The model under review builds one solid part; all positions refer to its coordinate system, in mm. A direction names the side the tool comes from. Coordinates: 2 decimals unless noted, no trailing zeros. Order: outer loops, then holes, each group sorted by start corner. A loop starts at its lowest first (then second) coordinate and runs counter-clockwise, first axis right, second up. Notation, with made-up numbers: M 13,-39.75 L 38,-39.75 A13 ccw 38,-18.75 Z; hole C -0.5,54 d2. An arc over 180 degrees is marked long. One line per item, written item: value.
```python
from build123d import *

# Parameters (mm, degrees)
MODEL_R             = 1.5
BOSS_EXTRUDE1_DEPTH = 6.6


with BuildPart() as part:
    # Model → Boss-Extrude1 (new body)
    with BuildSketch(Plane.XY):
        with BuildLine():
            Line((3.085786438, -24.814213562), (21.914213562, -5.985786438))
            ThreePointArc((21.914213562, -5.985786438), (22.347759065, -5.33693974), (22.5, -4.571572875))
            Line((22.5, -4.571572875), (22.5, 4.571572875))
            ThreePointArc((22.5, 4.571572875), (22.347759065, 5.33693974), (21.914213562, 5.985786438))
            Line((21.914213562, 5.985786438), (3.085786438, 24.814213562))
            ThreePointArc((3.085786438, 24.814213562), (2.43693974, 25.247759065), (1.671572875, 25.4))
            Line((1.671572875, 25.4), (-16.243953329, 25.4))
            ThreePointArc((-16.243953329, 25.4), (-20.102984306, 23.579289217), (-21.151543558, 19.44315197))
            ThreePointArc((-21.151543558, 19.44315197), (-19.273776994, 0), (-21.151543558, -19.44315197))
            ThreePointArc((-21.151543558, -19.44315197), (-20.102984306, -23.579289217), (-16.243953329, -25.4))
            Line((-16.243953329, -25.4), (1.671572875, -25.4))
            ThreePointArc((1.671572875, -25.4), (2.43693974, -25.247759065), (3.085786438, -24.814213562))
        make_face()
        with Locations((0.385786438, 20.4)):
            Circle(MODEL_R, mode=Mode.SUBTRACT)
        with Locations((0.385786438, -20.4)):
            Circle(MODEL_R, mode=Mode.SUBTRACT)
        with Locations((-7.922562904, 18.5)):
            Circle(MODEL_R, mode=Mode.SUBTRACT)
        with Locations((-7.899139633, -18.5)):
            Circle(MODEL_R, mode=Mode.SUBTRACT)
        with BuildLine():
            Line((-7.5, -2.5527), (7.5, -2.5527))
            ThreePointArc((7.5, -2.5527), (10.0527, 0), (7.5, 2.5527))
            Line((7.5, 2.5527), (-7.5, 2.5527))
            ThreePointArc((-7.5, 2.5527), (-10.0527, 0), (-7.5, -2.5527))
        make_face(mode=Mode.SUBTRACT)
    extrude(amount=BOSS_EXTRUDE1_DEPTH)


solid = part.part
```
(1) We need section D-D, the plane x = 19. State the section outline as (y, z) points.
Geometry results:
outline: M -8.9,0 L 8.9,0 L 8.9,6.6 L -8.9,6.6 Z
(2) Tool access review of faces 1 (the flat face through (0, -2.553, 3)), 2 (the cylindrical face through (-19.274, 0.274, 3.254)): name each direction out of +Z, -Z, +X, -X, +Y, -Y from which nothing blocks a thin tool from reaching the whole face with its end or side.
Geometry results:
face 1: +Z, -Z
face 2: +Z, -Z, -X
(3) Insertion check: pin 1 Ø2 at (y, z) = (-2, 3) entering from -X; pin 2 Ø3 at (x, z) = (12, 5) entering from +Y; pin 3 Ø3 at (y, z) = (-19, 1.5) entering from +X. Each pin has a flat end and moves straight along its axis. Give the tip position at first contact, or say it passes through.
Geometry results:
pin 1: stops at x = -19.32
pin 2: stops at y = 17.4
pin 3: stops at x = 10.4
(4) Mouldability with a two-part tool opening along X and no side actions: class faces 3 (the flat face through (-7, -25.4, 3)), 4 (the cylindrical face through (2.447, 25.244, 3.254)), 5 (the cylindrical face through (-20.142, -23.531, 3.254)), 6 (the cylindrical face through (-0.72, 21.414, 3.254)) as +X half, -X half, draft (parallel to the pull), parting line (faces both ways), or undercut.
Geometry results:
face 3: draft
face 4: +X half
face 5: -X half
face 6: undercut
(5) We need section C-C, the plane z = 0.75. State the section outline as (x, y) points, plus the area to 3 significant figures.
Geometry results:
outline: M -21.15,-19.44 A5 ccw -16.24,-25.4 L 1.67,-25.4 A2 ccw 3.09,-24.81 L 21.91,-5.99 A2 ccw 22.5,-4.57 L 22.5,4.57 A2 ccw 21.91,5.99 L 3.09,24.81 A2 ccw 1.67,25.4 L -16.24,25.4 A5 ccw -21.15,19.44 A101.6 cw Z; hole C -7.92,18.5 d3; hole C -7.9,-18.5 d3; hole M -7.5,-2.55 L 7.5,-2.55 A2.55 ccw 7.5,2.55 L -7.5,2.55 A2.55 ccw Z; hole C 0.39,-20.4 d3; hole C 0.39,20.4 d3
area: 1,630 mm2
(6) For L1, parallel to Y at x = 6, z = 1.75; L2, parallel to X at y = 19.5, z = 0.75; L3, parallel to Y at x = -7.5, z = 1.5, list the stretches that pass through material, from the lowest coordinate up.
Geometry results:
L1: y = -21.9 to -2.55, 2.55 to 21.9
L2: x = -21.16 to -9.04, -6.8 to -0.81, 1.59 to 8.4
L3: y = -25.4 to -19.95, -17.05 to -2.55, 2.55 to 17.06, 19.94 to 25.4
(7) We need section B-B, the plane x = 6.5. State the section outline as (y, z) points.
Geometry results:
outline: M -21.4,0 L -2.55,0 L -2.55,6.6 L -21.4,6.6 Z; M 2.55,0 L 21.4,0 L 21.4,6.6 L 2.55,6.6 Z
(8) We need section A-A, the plane y = 0. State the section outline as (x, z) points.
Geometry results:
outline: M -19.27,0 L -10.05,0 L -10.05,6.6 L -19.27,6.6 Z; M 10.05,0 L 22.5,0 L 22.5,6.6 L 10.05,6.6 Z
